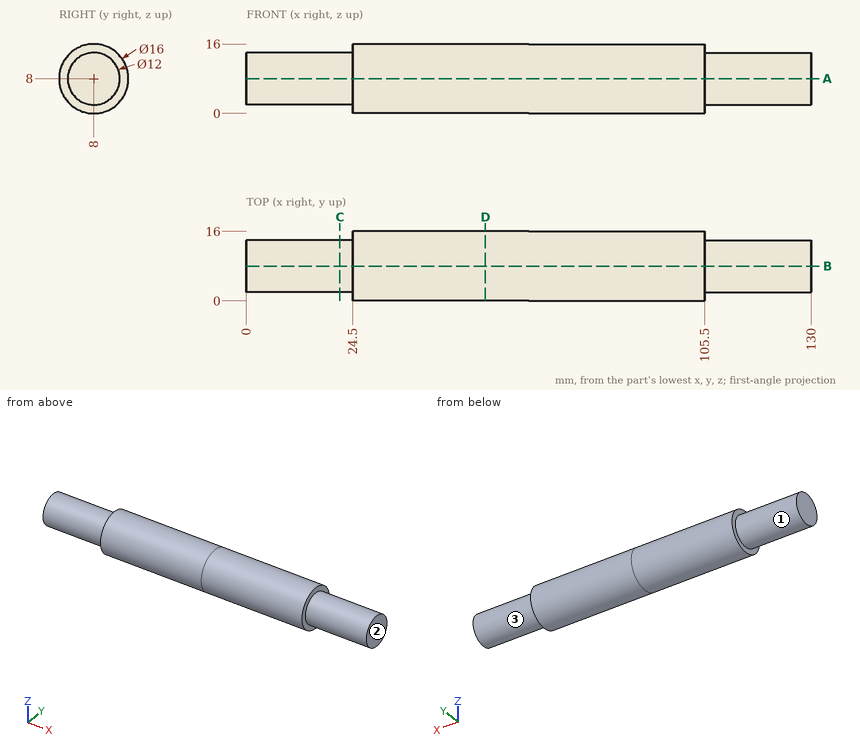
Part print with two shaded views. Sizes in mm from the minimum x, y, z corner. A direction names the side the tool comes from. Round coordinates to 2 decimals unless told otherwise and drop trailing zeros. Write each loop counter-clockwise with the first axis right and the second up, starting at its lowest first coordinate (ties: lowest second). Pieces come first, ordered by that corner, then holes. Notation, with made-up numbers: M -10,10 L 5,10 A11 ccw 5,17 Z; hole C 60,69.25 d9. An arc over 180 degrees is marked long. Put each result on its own line as item: value. Start each with the question number.
1) Saw through at D-D, the plane x = 55. Write the cut outline in (y, z).
2) Saw through at C-C, the plane x = 21.5. Write the cut outline in (y, z).
3) 3-axis set-ups, long thin cutter, end or side, ignore diameter. For the marked faces 1, 2 and 3: which of +Z, -Z, +X, -X, +Y, -Y reach the whole face in a straight line?
4) Drill centre lines: probe 1 along X at (y, z) = (5, 2); probe 2 along Y at (x, z) = (41, 8.5); probe 3 along Y at (x, z) = (42, 6). Where is each one in solid material? Low to high. Write a range as [from, to].
5) Saw through at A-A, the plane z = 8. Write the cut outline in (x, y), and give its area (3 significant figures).
6) Pin check, flat tips, straight feed: pin 1 Ø3 at (x, y) = (96, 3) entering from -Z; pin 2 Ø1 at (x, z) = (49, 3) entering from -Y; pin 3 Ø8 at (y, z) = (6, 8.5) entering from -X; pin 4 Ø3 at (x, y) = (19, 13.5) entering from +Z. Stop position of each tip, or through.
Resolved:
1. outline: C 8,8 d16
2. outline: C 8,8 d12
3. face 1: -X
3. face 2: +Z, -Z, +X, +Y, -Y
3. face 3: +X
4. probe 1: [24.5, 105.5]
4. probe 2: [0.02, 15.98]
4. probe 3: [0.25, 15.75]
5. outline: M 0,2 L 24.5,2 L 24.5,0 L 105.5,0 L 105.5,2 L 130,2 L 130,14 L 105.5,14 L 105.5,16 L 24.5,16 L 24.5,14 L 0,14 Z
5. area: 1,880 mm²
6. pin 1: z = 0.81
6. pin 2: y = 1.39
6. pin 3: x = 0
6. pin 4: z = 12.47
